from build123d import *

# Parameters (mm, degrees)
BOSS_EXTRUDE1_DEPTH = 19
SKETCH2_W           = 2.5
SKETCH2_H           = 2.5
CUT_EXTRUDE1_DEPTH  = 3
FILLET1_R           = 0.3


with BuildPart() as part:
    # Sketch1 → Boss-Extrude1 (new body)
    with BuildSketch(Plane(origin=(0, 0, 0), x_dir=(1, 0, 0), z_dir=(0, 1, 0))):
        with BuildLine():
            Line((8, -6), (8, 6))
            ThreePointArc((8, 6), (0, 10), (-8, 6))
            Line((-8, 6), (-8, -6))
            ThreePointArc((-8, -6), (0, -10), (8, -6))
        make_face()
    extrude(amount=BOSS_EXTRUDE1_DEPTH)

    # Sketch2 → Cut-Extrude1 (cut)
    with BuildSketch(Plane(origin=(0, 19, 0), x_dir=(1, 0, 0), z_dir=(0, 1, 0))):
        with Locations((0, -10)):
            Rectangle(SKETCH2_W, SKETCH2_H)
    cut_extrude1 = extrude(amount=-CUT_EXTRUDE1_DEPTH, mode=Mode.SUBTRACT)

    # Mirror1: Cut-Extrude1 across plane
    add(cut_extrude1.mirror(Plane.XY), mode=Mode.SUBTRACT)

    # Fillet1
    fillet1_edges = [part.edges().sort_by_distance(p)[0] for p in [
        (1.25, 17.5, 8.75),
        (0, 16, 8.75),
        (-1.25, 17.5, 8.75),
        (0, 16, -8.75),
        (-1.25, 17.5, -8.75),
        (1.25, 17.5, -8.75),
    ]]
    fillet(fillet1_edges, radius=FILLET1_R)


solid = part.part
Model file for the job. Use its own axes, mm. A direction names the side the tool comes from. Round coordinates to 2 decimals unless told otherwise and drop trailing zeros. Order: outer loops, then holes, each group sorted by start corner. A loop starts at its lowest first (then second) coordinate and runs counter-clockwise, first axis right, second up.
(1) Band-saw the part on D-D (y = 8.75). List the corners of the cut face in (x, z), then the cut area to 3 significant figures.
(2) Band-saw the part on A-A (x = 0). List the corners of the cut face in (y, z).
(3) Band-saw the part on C-C (z = -7.5). List the corners of the cut face in (x, y), then the cut area to 3 significant figures.
(4) Drill centre lines: line 1 (Z direction, x = -0.75, y = 16.75); line 2 (Z direction, x = 7.25, y = 15); line 3 (X direction, y = 12.25, z = -7.5). Where is each one in solid material? Low to high.
(5) Pull direction X, two halves, no side cores. Call faces 1 (the face through (8, 9, 0)), 2 (the face through (-1.25, 17.5, -9.5)), 3 (the face through (-8, 9, 0)), 4 (the face through (0, 9, 10)): released by +X, released by -X, zero draft, split by the parting line, or undercut.
(6) 3-axis set-ups, long thin cutter, end or side, ignore diameter. For faces 5 (the face through (1.25, 17.5, 9.5)), 6 (the face through (1.25, 17.5, -9.5)), 7 (the face through (0, 9, -10)): which of +Z, -Z, +X, -X, +Y, -Y reach the whole face in a straight line?
(7) Band-saw the part on B-B (y = 17.5). List the corners of the cut face in (x, z), then the cut area to 3 significant figures.
(8) Pin check, flat tips, straight feed: pin 1 (1 mm diameter, centred on x = -3.5, y = 15.5, fed in from +Z); pin 2 (1.5 mm diameter, centred on x = 0, y = 17.5, fed in from -Z); pin 3 (2 mm diameter, centred on x = 0, y = 18, fed in from +Z). Stop position of each tip, or through.
Verdict:
1. outline: (-8, -6) arc R10 ccw to (8, -6) - (8, 6) arc R10 ccw to (-8, 6) - close
1. area: 281 mm2
2. outline: (0, -10) - (16, -10) - (16, -9.05) arc R0.3 cw to (16.3, -8.75) - (19, -8.75) - (19, 8.75) - (16.3, 8.75) arc R0.3 cw to (16, 9.05) - (16, 10) - (0, 10) - close
3. outline: (-6.61, 0) - (6.61, 0) - (6.61, 19) - (-6.61, 19) - close
3. area: 251 mm2
4. line 1: z = -8.75 to 8.75
4. line 2: z = -6.89 to 6.89
4. line 3: x = -6.61 to 6.61
5. face 1: released by +X
5. face 2: undercut
5. face 3: released by -X
5. face 4: split by the parting line
6. face 5: +Z, +Y
6. face 6: -Z, +Y
6. face 7: -Z, +Y, -Y
7. outline: (-8, -6) arc R10 ccw to (-1.25, -9.92) - (-1.25, -9.05) arc R0.3 cw to (-0.95, -8.75) - (0.95, -8.75) arc R0.3 cw to (1.25, -9.05) - (1.25, -9.92) arc R10 ccw to (8, -6) - (8, 6) arc R10 ccw to (1.25, 9.92) - (1.25, 9.05) arc R0.3 cw to (0.95, 8.75) - (-0.95, 8.75) arc R0.3 cw to (-1.25, 9.05) - (-1.25, 9.92) arc R10 ccw to (-8, 6) - close
7. area: 275 mm2
8. pin 1: stops at z = 9.54
8. pin 2: stops at z = -8.75
8. pin 3: stops at z = 8.75
